```python
from build123d import *

# Parameters (mm, degrees)
SKETCH1_W           = 900
SKETCH1_H           = 375
BOSS_EXTRUDE1_DEPTH = 4
SKETCH2_W           = 900
SKETCH2_H           = 4
BOSS_EXTRUDE2_DEPTH = 80
SKETCH3_R           = 15
CUT_EXTRUDE1_DEPTH  = 80
CUT_EXTRUDE2_DEPTH  = 48


with BuildPart() as part:
    # Sketch1 → Boss-Extrude1 (new body)
    with BuildSketch(Plane(origin=(0, 0, 0), x_dir=(1, 0, 0), z_dir=(0, 1, 0))):
        Rectangle(SKETCH1_W, SKETCH1_H)
    extrude(amount=BOSS_EXTRUDE1_DEPTH)

    # Sketch2 → Boss-Extrude2 (add)
    with BuildSketch(Plane(origin=(0, 4, 0), x_dir=(1, 0, 0), z_dir=(0, 1, 0))):
        with Locations((0, -185.5)):
            Rectangle(SKETCH2_W, SKETCH2_H)
    extrude(amount=BOSS_EXTRUDE2_DEPTH)

    # Sketch3 → Cut-Extrude1 (cut)
    with BuildSketch(Plane(origin=(0, 4, 0), x_dir=(1, 0, 0), z_dir=(0, 1, 0))):
        with Locations(Location((375, 116.5, 0), (0, 0, 270))):
            Circle(SKETCH3_R)
        with Locations(Location((-375, 116.5, 0), (0, 0, 270))):
            Circle(SKETCH3_R)
    extrude(amount=-CUT_EXTRUDE1_DEPTH, mode=Mode.SUBTRACT)

    # Sketch6 → Cut-Extrude2 (cut)
    with BuildSketch(Plane(origin=(0, 30, 0), x_dir=(-1, 0, 0), z_dir=(0, -1, 0))):
        Polygon((375.476662109, 116.274639687), (375.476662109, 127.286348112), (343.747335513, 127.286348112), (343.747335513, 105.528943218), (375.476662109, 105.528943218), align=None)
    extrude(amount=CUT_EXTRUDE2_DEPTH, mode=Mode.SUBTRACT)


solid = part.part
```
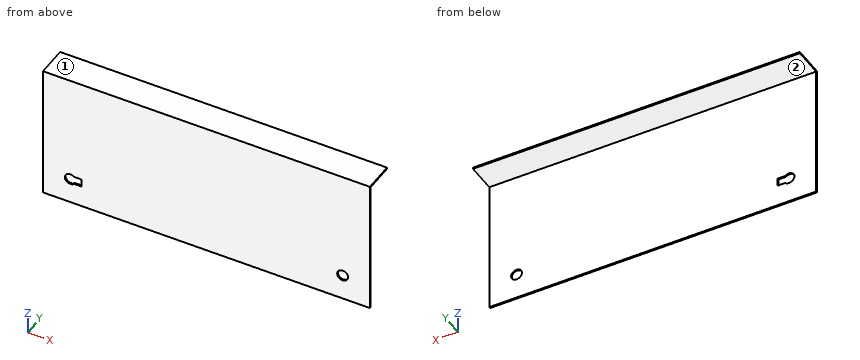
Can you work these out from the model? Positions are in its coordinate system, mm. Face numbers are marked on the shaded views. A direction names the side the tool comes from. Coordinates: 2 decimals unless noted, no trailing zeros. Loops run counter-clockwise (first coordinate to the right, second up) from the corner with the lowest first, then second, coordinate; pieces in that order, holes last.
Item 1: Suppose I cut it at B-B (x = 375). Please give me the cut outline in (y, z).
Answers below:
outline: (0, -187.5) - (4, -187.5) - (4, -131.5) - (0, -131.5) - close; (0, -101.5) - (4, -101.5) - (4, 183.5) - (84, 183.5) - (84, 187.5) - (0, 187.5) - close
Item 2: Suppose I cut it at D-D (x = -2). Please give me the cut outline in (y, z), then the cut area to 3 significant figures.
Answers below:
outline: (0, -187.5) - (4, -187.5) - (4, 183.5) - (84, 183.5) - (84, 187.5) - (0, 187.5) - close
area: 1,820 mm2
Item 3: Please list where these lines run through material, in increasing order: L1, parallel to X at y = 1.3, z = -116.5; L2, parallel to Z at x = -375, y = 2; L3, parallel to Y at x = 229, z = -60.
Answers below:
L1: x = -450 to -390, -343.75 to 360, 390 to 450
L2: z = -187.5 to -131.5, -101.5 to 187.5
L3: y = 0 to 4
Item 4: Suppose I cut it at A-A (z = -116.5). Please give me the cut outline in (x, y), then the cut area to 3 significant figures.
Answers below:
outline: (-450, 0) - (-390, 0) - (-390, 4) - (-450, 4) - close; (-343.75, 0) - (360, 0) - (360, 4) - (-343.75, 4) - close; (390, 0) - (450, 0) - (450, 4) - (390, 4) - close
area: 3,290 mm2
Item 5: I'm going to push flat-ended pins straight in: pin 1 (8 mm diameter, centred on x = 354, z = -22.5, fed in from +Y); pin 2 (6 mm diameter, centred on x = 18.5, y = 17.5, fed in from -Z). Where does each tip first touch, or does it pass through?
Answers below:
pin 1: stops at y = 4
pin 2: stops at z = 183.5
Item 6: Which directions (+Z, -Z, +X, -X, +Y, -Y) give clear straight access to the entire face, cutting with the end or side of a thin tool? Please do the marked faces 1 and 2.
Answers below:
face 1: +Z, +X, -X, +Y, -Y
face 2: -Z, +X, -X, +Y
Item 7: Suppose I cut it at C-C (y = 58.5). Please give me the cut outline in (x, z).
Answers below:
outline: (-450, 183.5) - (450, 183.5) - (450, 187.5) - (-450, 187.5) - close
